```python
from build123d import *

# Parameters (mm, degrees)
F0_R     = 22.86
F0_R_2   = 5.99948
F1_DEPTH = 7.9375


with BuildPart() as f1:
    # F0 (on Right) → F1 (new body, symmetric)
    with BuildSketch(Plane.YZ):
        Circle(F0_R)
        Circle(F0_R_2, mode=Mode.SUBTRACT)
    extrude(amount=F1_DEPTH, both=True)

    # F3: sweep along a path in F3_path
    with BuildLine(Plane(origin=(7.9375, 22.86, 0), x_dir=(0, 0, -1), z_dir=(-1, 0, 0))) as f3_path:
        CenterArc((0, 22.86), 22.86, 0, 360)
    # F2 (on Top) → F3 (sweep, cut)
    with BuildSketch(Plane.XY):
        Polygon((-4.1148, -22.86), (-7.9375, -19.0373), (-7.9375, -22.86), align=None)
        Polygon((-0.1524, -19.2024), (-3.81, -22.86), (3.81, -22.86), (0.1524, -19.2024), (0.1524, -19.0102346241), (0.0172294403, -19.0102346241), (-0.0172294403, -19.0102346241), (-0.1524, -19.0102346241), align=None)
        Polygon((7.9375, -19.0373), (4.1148, -22.86), (7.9375, -22.86), align=None)
    sweep(path=f3_path.line, mode=Mode.SUBTRACT)


solid = f1.part
```
Could you check a few things on this model? Use its own coordinates, in mm. A direction names the side the tool comes from. Round coordinates to 2 decimals unless told otherwise and drop trailing zeros. Loops run counter-clockwise (first coordinate to the right, second up) from the corner with the lowest first, then second, coordinate; pieces in that order, holes last. Notation, with made-up numbers: (-38.75, -19.5) - (-22.75, -19.5) arc R20 cw to (-22.75, 12.5) - close; hole circle Ø3 at (-29.75, -5). An arc over 180 degrees is marked (long way). Answer in a Markdown table with one row per item. Add a question column.
(1) If we section it at A-A (x = 6.5): Please give me the cut outline in (y, z), plus the area to 3 significant figures.
(2) I'm going to push flat-ended pins straight in: pin 1 (3 mm diameter, centred on x = 4.5, y = -5.5, fed in from -Z); pin 2 (8 mm diameter, centred on x = 0, z = -11.5, fed in from -Y); pin 3 (3 mm diameter, centred on x = -6, z = -13.5, fed in from +Y). Where does each tip first touch, or does it pass through?
(3) If we mould it in two halves opening along X, with no side actions, what happens to faces 1 (the face through (7.698, -5.79, -18.386)), 2 (the face through (-0.11, -0.78, 5.95)), 3 (the face through (-0.38, -16.38, -10.45))? For each: pulls with the +X half, pulls with the -X half, needs draft (parallel to the pull), parting line crosses it, or undercut.
(4) If we section it at B-B (x = 1.25): Please give me the cut outline in (y, z), plus the area to 3 significant figures.
(5) For faces 4 (the face through (0, 18.56, 4.12)), 5 (the face through (-7.938, -4.5, 4.5)), which set-ups out of +Z, -Z, +X, -X, +Y, -Y let a thin tool reach every point of the face, with its end or its side?
(6) I need wall thicknesses on line 1 along Y through (x, z) = (1, 4.5); line 2 along Z through (x, y) = (-0.25, 0); line 3 along Z through (x, y) = (2.25, 0). Which ranges of each line are inside material? Lowest first, please.
Model answer:
| question | item | result |
|---|---|---|
| 1 | outline | circle Ø40.95 at (0, 0); hole circle Ø12 at (0, 0) |
| 1 | area | 1,200 mm² |
| 2 | pin 1 | stops at z = -22.5 |
| 2 | pin 2 | stops at y = -20.45 |
| 2 | pin 3 | stops at y = 18.26 |
| 3 | face 1 | pulls with the +X half |
| 3 | face 2 | needs draft |
| 3 | face 3 | undercut |
| 4 | outline | circle Ø40.6 at (0, 0); hole circle Ø12 at (0, 0) |
| 4 | area | 1,180 mm² |
| 5 | face 4 | none |
| 5 | face 5 | +Z, -Z, -X, +Y, -Y |
| 6 | line 1 | y = -19.54 to -3.97, 3.97 to 19.54 |
| 6 | line 2 | z = -19.3 to -6, 6 to 19.3 |
| 6 | line 3 | z = -21.3 to -6, 6 to 21.3 |
